Work out the finished part from the listing and answer in its coordinate system (mm). Face numbers are marked on the shaded views. A direction names the side the tool comes from. Coordinates: 2 decimals unless noted, no trailing zeros. One line per item, written item: value.
```python
from build123d import *

# Parameters (mm, degrees)
SKETCH1_W            = 23.8125
SKETCH1_H            = 15.875
BASE_EXTRUDE_DEPTH   = 9.525
SKETCH2_R            = 2.4384
BOSS_EXTRUDE1_DEPTH  = 1.905
LPATTERN4_COUNT      = 3
LPATTERN4_PITCH      = 7.9375
LPATTERN4_COUNT_DIR2 = 2
LPATTERN4_PITCH_DIR2 = 7.9375
CUT_EXTRUDE1_DEPTH   = 23.900203363
SHELL1_T             = -1.5875
INSDOT_REACH         = 20.314
SKETCH3_R            = 3.2004
SKETCH3_R_2          = 2.4384
LPATTERN5_COUNT      = 2
LPATTERN5_PITCH      = 7.9375
FILLET1_R            = 0.254


with BuildPart() as part:
    # Sketch1 → Base-Extrude (new body)
    with BuildSketch(Plane(origin=(0, 0, 0), x_dir=(1, 0, 0), z_dir=(0, 1, 0))):
        Rectangle(SKETCH1_W, SKETCH1_H)
    extrude(amount=BASE_EXTRUDE_DEPTH)

    # Sketch2 → Boss-Extrude1 (add)
    with BuildSketch(Plane(origin=(0, 9.525, 0), x_dir=(-1, 0, 0), z_dir=(0, 1, 0))):
        with Locations(Location((7.9375, 3.96875, 0), (0, 0, 270))):
            Circle(SKETCH2_R)
    boss_extrude1 = extrude(amount=BOSS_EXTRUDE1_DEPTH)

    # LPattern4: Boss-Extrude1 3 × 2
    with Locations(*[(i * LPATTERN4_PITCH, 0, -j * LPATTERN4_PITCH_DIR2) for i in range(LPATTERN4_COUNT) for j in range(LPATTERN4_COUNT_DIR2) if (i, j) != (0, 0)]):
        add(boss_extrude1)

    # Sketch4 → Cut-Extrude1 (cut, through all)
    with BuildSketch(Plane.XY.offset(7.9375)):
        Polygon((-3.96875, 9.525), (11.90625, 2.159), (11.90625, 11.43), (-3.96875, 11.43), align=None)
    extrude(amount=-CUT_EXTRUDE1_DEPTH, mode=Mode.SUBTRACT)

    # Shell1
    shell1_openings = [part.faces().sort_by_distance(p)[0] for p in [
        (0, 0, 0),
    ]]
    offset(amount=SHELL1_T, openings=shell1_openings, kind=Kind.INTERSECTION)

    # Sketch3 → InsDot (add, up to next)
    with BuildSketch(Plane.XZ, mode=Mode.PRIVATE) as insdot_sk1:
        with Locations((-3.96875, 0)):
            Circle(SKETCH3_R)
        with Locations((-3.96875, 0)):
            Circle(SKETCH3_R_2, mode=Mode.SUBTRACT)
    insdot_tool1 = extrude(insdot_sk1.sketch, amount=-INSDOT_REACH, mode=Mode.PRIVATE) - part.part
    insdot = insdot_tool1.solids().sort_by_distance((-7.078629, 0, 0))[0]
    add(insdot)

    # LPattern5: InsDot; each copy of InsDot runs up to whatever stops it at its own place
    lpattern5_before = part.part  # the part as the pattern finds it: every copy runs up to it
    lpattern5_insdot_long = extrude(insdot_sk1.sketch, amount=-INSDOT_REACH, mode=Mode.PRIVATE)
    lpattern5_insdot_tool1 = lpattern5_insdot_long.moved(Location(Vector(1, 0, 0) * (1 * LPATTERN5_PITCH))) - lpattern5_before
    add(lpattern5_insdot_tool1.solids().sort_by_distance((0.858871, 0, 0))[0])

    # Fillet1
    fillet1_edges = [part.edges().sort_by_distance(p)[0] for p in [
        (-7.9375, 9.525, -7.9375),
        (-7.9375, 9.525, 7.9375),
        (3.96875, 5.842, 7.9375),
        (-3.96875, 9.525, 0),
        (3.96875, 5.842, -7.9375),
        (11.90625, 2.159, 0),
        (-11.90625, 9.525, 0),
    ]]
    fillet(fillet1_edges, radius=FILLET1_R)


solid = part.part
```
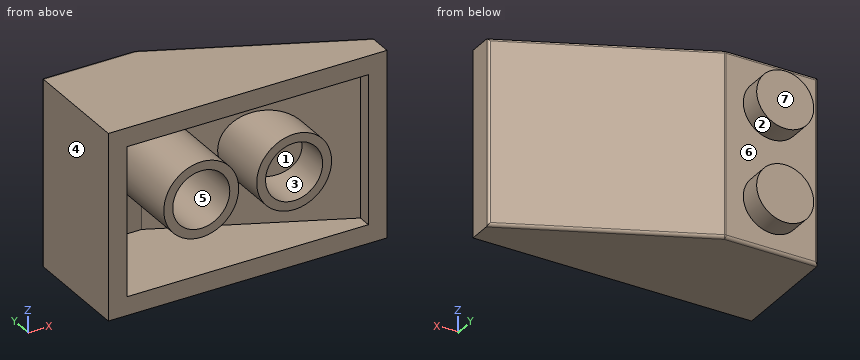
Item 1: Consider probe 1 along Z at (x, y) = (9.75, 1.25); probe 2 along X at (y, z) = (4, 1.5). Determine where each line is inside the solid, lowest interval first.
Evaluation:
probe 1: z = -7.94 to -6.35, 6.35 to 7.94
probe 2: x = -11.91 to -10.32, -6.8 to -5.89, -2.05 to -1.14, 1.14 to 2.05, 4.17 to 7.94
Item 2: Determine the mould class of the marked faces 1, 2, 3 and 4 for opening direction X: +X half, -X half, draft (parallel to the pull), parting line (faces both ways), or undercut.
Evaluation:
face 1: undercut
face 2: parting line
face 3: undercut
face 4: -X half
Item 3: Which of the six approach directions +Z, -Z, +X, -X, +Y, -Y give full straight-line access (tool end or side, diameter ignored) to the marked faces 5, 6 and 7?
Evaluation:
face 5: -Y
face 6: +Y
face 7: +Z, -Z, +X, -X, +Y
Item 4: Given pin 1 (1 mm diameter, centred on y = 8.5, z = -3, fed in from +X); pin 2 (1.9 mm diameter, centred on x = -8, z = -3.5, fed in from -Y); pin 3 (4 mm diameter, centred on x = -3.97, z = 0, fed in from +Y) (3 decimals), each flat-ended and moving along its own axis, determine where each tip first touches the part or whether it passes through.
Evaluation:
pin 1: stops at x = -0.68
pin 2: stops at y = 7.94
pin 3: stops at y = 9.525
Item 5: Section C-C, the plane y = 6 is taken. Give the number of separate pieces and of enclosed holes in the cut face, then the cut area to 3 significant figures.
Evaluation:
separate pieces: 2
enclosed holes: 2
area: 131 mm2
